from build123d import *

# Parameters (mm, degrees)
F1_DEPTH = 25


with BuildPart() as f1:
    # F0 (on Front) → F1 (new body)
    with BuildSketch(Plane.XZ):
        with BuildLine():
            Line((29, 33.451155), (-31.5, 33.451155))
            ThreePointArc((-31.5, 33.451155), (-32.56066, 33.011816), (-33, 31.951155))
            Line((-33, 31.951155), (-33, 30.451155))
            Line((-33, 30.451155), (-3, 30.451155))
            Line((-3, 30.451155), (-3, -4.748845))
            Line((-3, -4.748845), (-42.949969, -2.748845))
            Line((-42.949969, -2.748845), (-42.949969, -4.327762))
            ThreePointArc((-42.949969, -4.327762), (-42.538887, -5.359391), (-41.530959, -5.825574))
            Line((-41.530959, -5.825574), (-2.107987, -7.957275))
            ThreePointArc((-2.107987, -7.957275), (-0.624495, -7.412083), (0, -5.960192))
            Line((0, -5.960192), (0, 28.451155))
            ThreePointArc((0, 28.451155), (0.585786, 29.865369), (2, 30.451155))
            Line((2, 30.451155), (31.5, 30.451155))
            ThreePointArc((31.5, 30.451155), (32.56066, 30.890495), (33, 31.951155))
            Line((33, 31.951155), (33, 36.951155))
            ThreePointArc((33, 36.951155), (32.56066, 38.011816), (31.5, 38.451155))
            ThreePointArc((31.5, 38.451155), (30.43934, 38.011816), (30, 36.951155))
            Line((30, 36.951155), (30, 34.451155))
            ThreePointArc((30, 34.451155), (29.707107, 33.744049), (29, 33.451155))
        make_face()
    extrude(amount=F1_DEPTH)


solid = f1.part
Build history of the part. All positions in model axes, mm. A direction names the side the tool comes from. Coordinates: 2 decimals unless noted, no trailing zeros. Write each loop counter-clockwise with the first axis right and the second up, starting at its lowest first coordinate (ties: lowest second). Pieces come first, ordered by that corner, then holes.
(1) Cut at A-A on x = -28. List the corners of the cut face in (y, z), and give its area (3 significant figures).
(2) Drill centre lines: line 1 (X direction, y = -9, z = 28); line 2 (Z direction, x = 11.5, y = -3.5); line 3 (Z direction, x = -22, y = -12.25). Where is each one in solid material? Low to high.
(3) Cut at B-B on y = -10. List the corners of the cut face in (x, z).
(4) Pin check, flat tips, straight feed: pin 1 Ø2 at (y, z) = (-9.5, 36.5) entering from -X; pin 2 Ø2 at (x, y) = (0.5, -9) entering from +Z; pin 3 Ø3 at (x, y) = (-15.5, -6.5) entering from -Z. Stop position of each tip, or through.
(5) 3-axis set-ups, long thin cutter, end or side, ignore diameter. For faces 1 (the flat face through (-22.695, -12.325, -3.763)), 2 (the flat face through (30, -12, 36)), 3 (the flat face through (-18, -12, 30.451)), 4 (the cylindrical face through (-42.55, -12.32, -5.35)), 5 (the flat face through (17, -12, 30.451)): which of +Z, -Z, +X, -X, +Y, -Y reach the whole face in a straight line?
(6) Cut at D-D on z = 23. List the corners of the cut face in (x, y), and give its area (3 significant figures).
(7) Cut at C-C on x = -7. List the corners of the cut face in (y, z), and give its area (3 significant figures).
Working result:
1. outline: (-25, -6.56) - (0, -6.56) - (0, -3.5) - (-25, -3.5) - close; (-25, 30.45) - (0, 30.45) - (0, 33.45) - (-25, 33.45) - close
1. area: 151 mm2
2. line 1: x = -3 to 0
2. line 2: z = 30.45 to 33.45
2. line 3: z = -6.88 to -3.8, 30.45 to 33.45
3. outline: (-42.95, -4.33) arc R1.5 ccw to (-41.53, -5.83) - (-2.11, -7.96) arc R2 ccw to (0, -5.96) - (0, 28.45) arc R2 cw to (2, 30.45) - (31.5, 30.45) arc R1.5 ccw to (33, 31.95) - (33, 36.95) arc R1.5 ccw to (31.5, 38.45) arc R1.5 ccw to (30, 36.95) - (30, 34.45) arc R1 cw to (29, 33.45) - (-31.5, 33.45) arc R1.5 ccw to (-33, 31.95) - (-33, 30.45) - (-3, 30.45) - (-3, -4.75) - (-42.95, -2.75) - close
4. pin 1: stops at x = 30
4. pin 2: stops at z = 33.45
4. pin 3: stops at z = -7.31
5. face 1: +Y, -Y
5. face 2: +Z, -X, +Y, -Y
5. face 3: -X, +Y, -Y
5. face 4: -Z, -X, +Y, -Y
5. face 5: -Z, +X, +Y, -Y
6. outline: (-3, -25) - (0, -25) - (0, 0) - (-3, 0) - close
6. area: 75.0 mm2
7. outline: (-25, -7.69) - (0, -7.69) - (0, -4.55) - (-25, -4.55) - close; (-25, 30.45) - (0, 30.45) - (0, 33.45) - (-25, 33.45) - close
7. area: 154 mm2
